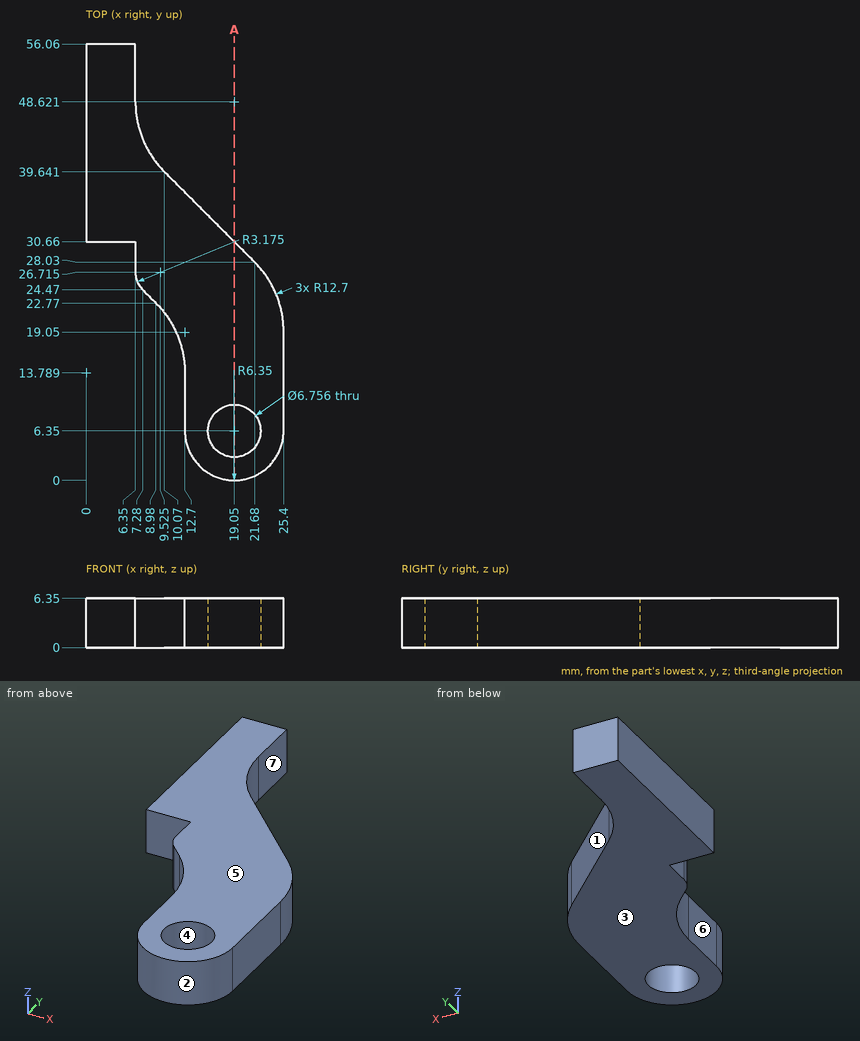
Job drawing, mm, ordinate dimensions from the low corner. One solid piece. A direction names the side the tool comes from. Give positions to 0.01 mm unless a question says otherwise; leave off trailing zeros. Loops run counter-clockwise (first coordinate to the right, second up) from the corner with the lowest first, then second, coordinate; pieces in that order, holes last. Notation, with made-up numbers: (-6.75, 57.25) -> (25.25, 57.25) arc R15 ccw to (25.25, 78.25) -> close; hole circle Ø9 at (85.25, -18.5). An arc over 180 degrees is marked (long way). Write each question's results on one line, items separated by ' | '.
(1) Tool access for the marked faces 5, 6 and 7: list every direction of +Z, -Z, +X, -X, +Y, -Y with a clear straight run to the whole face (end or side of a thin tool).
Geometry results:
face 5: +Z, +X, -X, +Y, -Y | face 6: +Z, -Z, -X, -Y | face 7: +Z, -Z, +X, +Y
(2) Cut at A-A on x = 19.05. List the corners of the cut face in (y, z).
Geometry results:
outline: (0, 0) -> (2.97, 0) -> (2.97, 6.35) -> (0, 6.35) -> close; (9.73, 0) -> (30.66, 0) -> (30.66, 6.35) -> (9.73, 6.35) -> close
(3) Probe line 1 along Y through (x, z) = (19.05, 1.5); line 2 along X through (y, z) = (6.35, 2.5); line 3 along Y through (x, z) = (5, 6.25). List the from-to ranges inside material, lowest first.
Geometry results:
line 1: y = 0 to 2.97, 9.73 to 30.66 | line 2: x = 12.7 to 15.67, 22.43 to 25.4 | line 3: y = 30.66 to 56.06
(4) Flat gauge pins, fed straight in: pin 1 Ø3 at (x, z) = (6, 4) entering from -Y; pin 2 Ø1.2 at (y, z) = (28.5, 3) entering from -X; pin 3 Ø8 at (x, y) = (13.5, 28) entering from -Z; pin 4 Ø3 at (x, z) = (1.5, 3.5) entering from -Y. Where does each tip first touch, or does it go through?
Geometry results:
pin 1: stops at y = 24.25 | pin 2: stops at x = 6.35 | pin 3: stops at z = 0 | pin 4: stops at y = 30.66
(5) Pull direction Y, two halves, no side cores. Call the marked faces 1, 2, 3 and 4: released by +Y, released by -Y, zero draft, split by the parting line, or undercut.
Geometry results:
face 1: released by +Y | face 2: released by -Y | face 3: zero draft | face 4: undercut
